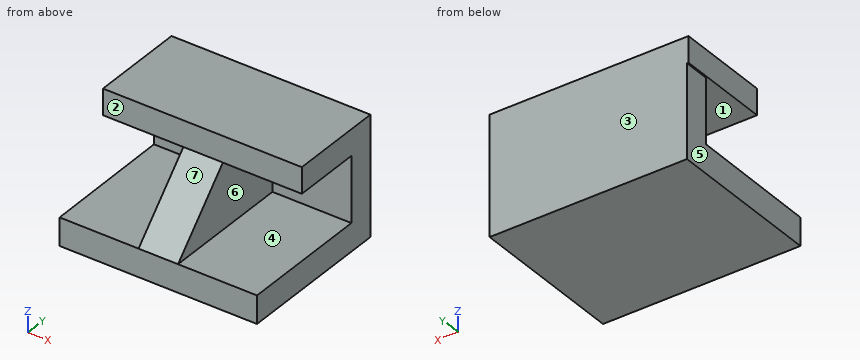
from build123d import *

# Parameters (mm, degrees)
F0_W      = 96.990541555
F0_H      = 38.3299775422
F1_DEPTH  = 50.8
F3_DEPTH  = 101.6
F5_DEPTH  = 25.4
F7_DEPTH  = 38.1
F8_DEPTH  = 38.1
F9_W      = 33.0152064562
F9_H      = 8.3422744647
F10_DEPTH = 47.752
F11_DEPTH = 25.4
F13_DEPTH = 25.4
F15_DEPTH = 63.5
F17_DEPTH = 25.4
F19_DEPTH = 25.4
F20_DEPTH = 9.906
F22_DEPTH = 25.4


# Not quite as in the source:
# - a feature of the source that left no trace in its solid (it failed there, or was rolled back) is left out


with BuildPart() as f1:
    # F0 (on Front) → F1 (new body)
    with BuildSketch(Plane.XZ):
        with Locations((-52.56479932, -19.1649887711)):
            Rectangle(F0_W, F0_H)
    extrude(amount=F1_DEPTH)

    # F2 (on face) → F3 (cut)
    with BuildSketch(Plane.YZ.offset(-4.0695285425)):
        Polygon((-50.8, 0), (-50.8, -29.3875597417), (-30.714739114, -8.3422744647), (-30.714739114, 0), align=None)
    extrude(amount=-F3_DEPTH, mode=Mode.SUBTRACT)

    # F4 (on face) → F5 (cut)
    with BuildSketch(Plane.YZ.offset(-4.0695285425)):
        Polygon((-8.5318721831, -8.3422744647), (-30.714739114, -8.3422744647), (-50.8, -29.3875597417), (-8.5318721831, -29.3875597417), align=None)
    extrude(amount=-F5_DEPTH, mode=Mode.SUBTRACT)

    # F6 (on face) → F7 (cut)
    with BuildSketch(Plane(origin=(-101.0600700974, 0, 0), x_dir=(0, -1, 0), z_dir=(-1, 0, 0))):
        Polygon((50.8, -29.3875597417), (30.714739114, -8.3422744647), (10.0486502051, -8.3422744647), (10.0486502051, -29.3875597417), align=None)
    extrude(amount=-F7_DEPTH, mode=Mode.SUBTRACT)

    # F8 (cut): a face of the model
    f8_faces = [f1.faces().sort_by_distance(p)[0] for p in [
        (-29.4695285425, -25.1662286777, -19.9579957719),
    ]]
    extrude(f8_faces, amount=-F8_DEPTH, mode=Mode.SUBTRACT)

    # F9 (on face) → F10 (cut)
    with BuildSketch(Plane.XZ.offset(30.714739114)):
        with Locations((-84.5524668694, -4.1711372323)):
            Rectangle(F9_W, F9_H)
    extrude(amount=-F10_DEPTH, mode=Mode.SUBTRACT)

    # F11 (cut): a face of the model
    f11_faces = [f1.faces().sort_by_distance(p)[0] for p in [
        (-84.31479932, -10.0486502051, -18.8649171032),
    ]]
    extrude(f11_faces, amount=-F11_DEPTH, mode=Mode.SUBTRACT)

    # F12 (on face) → F13 (cut)
    with BuildSketch(Plane.XY.offset(-29.3875597417)):
        Polygon((-67.5695285425, -50.8), (-67.5695285425, -8.5318721831), (-67.5695285425, 0), (-101.0600700974, 0), (-101.0600700974, -50.8), align=None)
    extrude(amount=-F13_DEPTH, mode=Mode.SUBTRACT)

    # F14 (on face) → F15 (join)
    with BuildSketch(Plane(origin=(-67.5695285425, 0, 0), x_dir=(0, -1, 0), z_dir=(-1, 0, 0))):
        Polygon((50.8, -29.3875597417), (8.5318721831, -8.3422744647), (8.5318721831, -29.3875597417), align=None)
    extrude(amount=-F15_DEPTH)

    # F16 (on face) → F17 (cut)
    with BuildSketch(Plane.YZ.offset(-4.0695285425)):
        Polygon((-8.5318721831, -8.3422744647), (-50.8, -29.3875597417), (-8.5095763206, -29.3875597417), align=None)
    extrude(amount=-F17_DEPTH, mode=Mode.SUBTRACT)

    # F18 (on face) → F19 (cut)
    with BuildSketch(Plane(origin=(-67.5695285425, 0, 0), x_dir=(0, -1, 0), z_dir=(-1, 0, 0))):
        Polygon((50.8, -29.3875597417), (8.5318721831, -8.3422744647), (8.5318721831, -29.1403066367), align=None)
    extrude(amount=-F19_DEPTH, mode=Mode.SUBTRACT)

    # F20 (add): a face of the model
    f20_faces = [f1.faces().sort_by_distance(p)[0] for p in [
        (-35.8195285425, -29.6659360915, -18.8649171032),
    ]]
    extrude(f20_faces, amount=F20_DEPTH)

    # F21 (on face) → F22 (cut)
    with BuildSketch(Plane.YZ.offset(-29.4695285425)):
        Polygon((-55.2151913765, -20.5199263986), (-50.8, -29.3875597417), (-30.714739114, -8.3211602381), align=None)
        Polygon((-12.9470635596, 0.5253588785), (-14.0022137243, 0), (-12.6854875674, 0), align=None)
    extrude(amount=-F22_DEPTH, mode=Mode.SUBTRACT)


solid = f1.part
Design review of the part built by this model. Coordinates are the model's own, in mm. Face numbers are marked on the shaded views. A direction names the side the tool comes from. Coordinates: 2 decimals unless noted, no trailing zeros. Write each loop counter-clockwise with the first axis right and the second up, starting at its lowest first coordinate (ties: lowest second). Pieces come first, ordered by that corner, then holes. Notation, with made-up numbers: (6, 56.5) - (50, 56.5) arc R25 cw to (50, 81.5) - close; hole circle Ø7 at (-8, -20). An arc over 180 degrees is marked (long way). Use one line per item in the form item = value.
Q1. Consider section B-B (y = -17.5). Write out the cut boundary in (x, z).
Taken from the geometry:
outline = (-68.04, -8.34) - (-42.17, -8.34) - (-42.17, -29.19) - (-67.57, -29.19) - (-67.57, -38.33) - (-4.07, -38.33) - (-4.07, -29.39) - (-29.47, -29.39) - (-29.47, -8.34) - (-4.07, -8.34) - (-4.07, 0) - (-68.04, 0) - close
Q2. Consider section A-A (x = -16). Write out the cut boundary in (y, z).
Taken from the geometry:
outline = (-50.8, -38.33) - (0, -38.33) - (0, 0) - (-30.71, 0) - (-30.71, -8.34) - (-8.53, -8.34) - (-8.51, -29.39) - (-50.8, -29.39) - close
Q3. Consider section D-D (y = -11.5). Write out the cut boundary in (x, z), plus the area to 3 significant figures.
Taken from the geometry:
outline = (-68.04, -8.34) - (-42.17, -8.34) - (-42.17, -29.16) - (-67.57, -29.16) - (-67.57, -38.33) - (-4.07, -38.33) - (-4.07, -29.39) - (-29.47, -29.39) - (-29.47, -8.34) - (-4.07, -8.34) - (-4.07, 0) - (-68.04, 0) - close
area = 1,370 mm^2
Q4. Consider section C-C (z = -14). Write out the cut boundary in (x, y), plus the area to 3 significant figures.
Taken from the geometry:
outline = (-67.57, -8.53) - (-42.17, -8.53) - (-42.17, -36.13) - (-29.47, -36.13) - (-29.47, -8.53) - (-4.07, -8.53) - (-4.07, 0) - (-67.57, 0) - close
area = 892 mm^2
Q5. Insertion check: pin 1 Ø3 at (x, y) = (-26, -33.5) entering from +Z; pin 2 Ø4 at (y, z) = (-38.5, -15.5) entering from -X; pin 3 Ø6.5 at (y, z) = (-38.5, -21.5) entering from +X. Each pin has a flat end and moves straight along its axis. Give the tip position at first contact, or say it passes through.
Taken from the geometry:
pin_1 = -29.39
pin_2 = -42.17
pin_3 = -29.47
Q6. For probe 1 along Z at (x, y) = (-7.5, -17); probe 2 along Y at (x, z) = (-11, -6); probe 3 along X at (y, z) = (-3.5, -30), list the stretches that pass through material, from the lowest coordinate up.
Taken from the geometry:
probe_1 = -38.33 to -29.39, -8.34 to 0
probe_2 = -30.71 to 0
probe_3 = -67.57 to -4.07
Q7. Machinability: for the marked faces 1, 2, 3 and 4, which of the approach directions +Z, -Z, +X, -X, +Y, -Y give a long, thin tool a straight path to every point of the face, cutting with its end or side? Answer none if there is none.
Taken from the geometry:
face_1 = -X, -Y
face_2 = +Z, +X, -X, -Y
face_3 = +Z, -Z, +X, -X, +Y
face_4 = +X, -Y
Q8. The part is to be moulded in two halves that separate along Z. For the marked faces 5, 6 and 7, say which applies: +Z half, -Z half, draft (parallel to the pull), parting line (faces both ways), or undercut.
Taken from the geometry:
face_5 = draft
face_6 = undercut
face_7 = +Z half
